The figure shows three views and two pictorial views of one solid part (mm, origin at its lowest corner). Answer the questions. Round coordinates to 2 decimals unless told otherwise and drop trailing zeros. Write each loop counter-clockwise with the first axis right and the second up, starting at its lowest first coordinate (ties: lowest second). Pieces come first, ordered by that corner, then holes.
Item 1: Find the intervals of material crossed by probe 1 along Z at (x, y) = (756.5, 32.5); probe 2 along Z at (x, y) = (735, 44), in increasing order.
Item 2: Find section A-A on y = 150.5. Give the vertices of the cut face in (x, z) (1 decimal).
Item 3: Find section B-B on z = 7.5. Give the vertices of the cut face in (x, y), then the cut area to 3 significant figures.
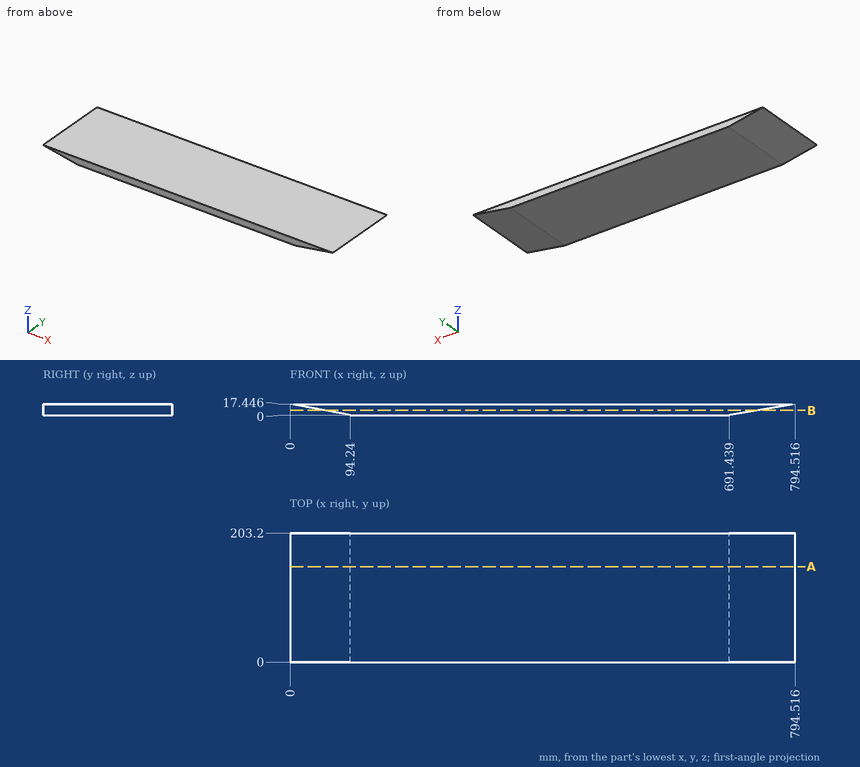
Check values:
1. probe 1: z = 11.01 to 17.45
1. probe 2: z = 7.37 to 17.45
2. outline: (0, 17.4) - (94.2, 0) - (691.4, 0) - (794.5, 17.4) - close
3. outline: (53.73, 0) - (735.75, 0) - (735.75, 203.2) - (53.73, 203.2) - close
3. area: 139,000 mm2
